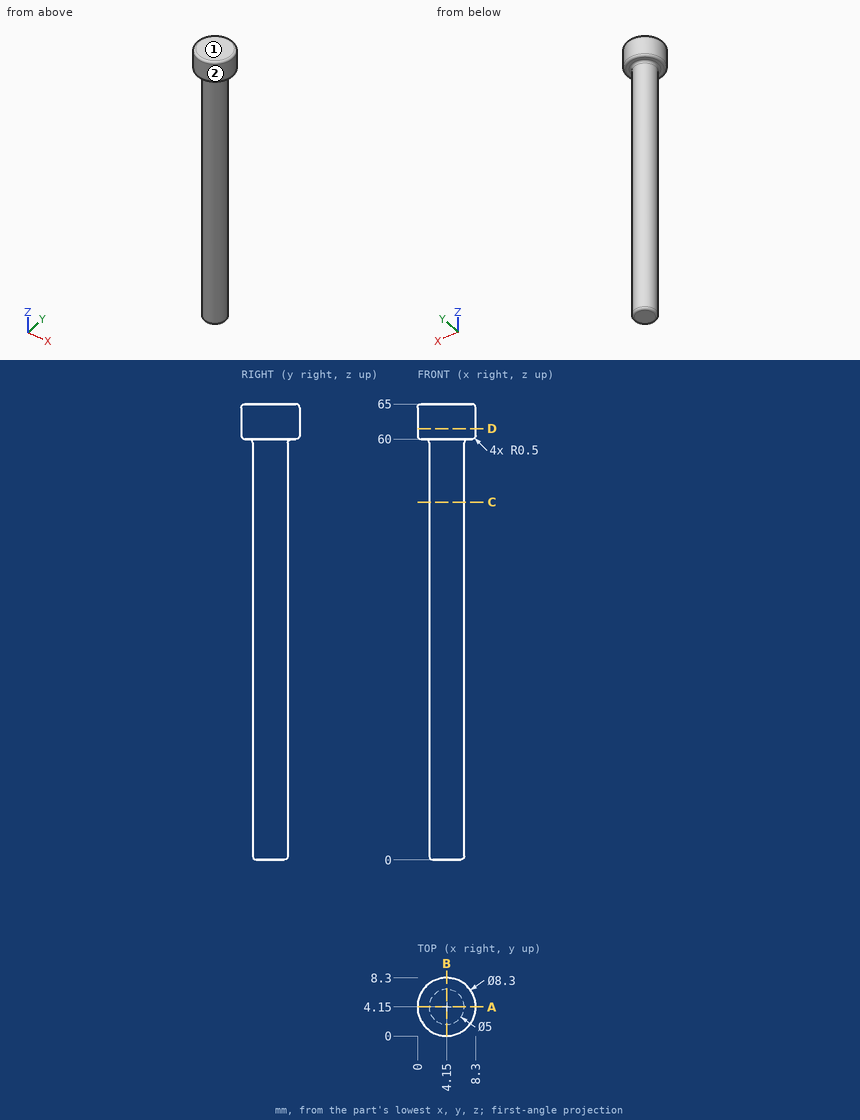
Print and shaded views of the part. All mm, measured from the part's lowest x, y and z. Coordinates: 2 decimals unless noted, no trailing zeros. Write each loop counter-clockwise with the first axis right and the second up, starting at its lowest first coordinate (ties: lowest second). Pieces come first, ordered by that corner, then holes. Notation, with made-up numbers: (-35.75, -33) -> (12.25, -33) arc R33 cw to (12.25, 1) -> close; hole circle Ø1 at (24.5, 79). An arc over 180 degrees is marked (long way). Use CSV: the item, a comma, the result in double quotes. Start each with the question number.
Q1. Drill centre lines: probe 1 along Z at (x, y) = (2.75, 7.5); probe 2 along X at (y, z) = (4, 20); probe 3 along X at (y, z) = (5.5, 20.5). Where is each one in solid material? Low to high.
Q2. Flat gauge pins, fed straight in: pin 1 Ø4 at (y, z) = (3, 42.5) entering from +X; pin 2 Ø2 at (x, z) = (4, 29.5) entering from -Y; pin 3 Ø4 at (y, z) = (7, 18.5) entering from -X. Where does each tip first touch, or does it go through?
Q3. Cut at C-C, the plane z = 51. List the corners of the cut face in (x, y), then the cut area to 3 significant figures.
Q4. Pull direction Z, two halves, no side cores. Call the marked faces 1 and 2: released by +Z, released by -Z, zero draft, split by the parting line, or undercut.
Q5. Cut at A-A, the plane y = 4.15. List the corners of the cut face in (x, z), then the cut area to 3 significant figures.
Q6. Cut at D-D, the plane z = 61.5. List the corners of the cut face in (x, y), then the cut area to 3 significant figures.
Checked values:
1,probe 1,"z = 60 to 65"
1,probe 2,"x = 1.65 to 6.65"
1,probe 3,"x = 2.05 to 6.25"
2,pin 1,"stops at x = 6.65"
2,pin 2,"stops at y = 1.65"
2,pin 3,"stops at x = 1.8"
3,outline,"circle Ø5 at (4.15, 4.15)"
3,area,"19.6 mm²"
4,face 1,"released by +Z"
4,face 2,"zero draft"
5,outline,"(0, 60.5) arc R0.5 ccw to (0.5, 60) -> (1.15, 60) arc R0.5 cw to (1.65, 59.5) -> (1.65, 0.5) arc R0.5 ccw to (2.15, 0) -> (6.15, 0) arc R0.5 ccw to (6.65, 0.5) -> (6.65, 59.5) arc R0.5 cw to (7.15, 60) -> (7.8, 60) arc R0.5 ccw to (8.3, 60.5) -> (8.3, 64.5) arc R0.5 ccw to (7.8, 65) -> (0.5, 65) arc R0.5 ccw to (0, 64.5) -> close"
5,area,"341 mm²"
6,outline,"circle Ø8.3 at (4.15, 4.15)"
6,area,"54.1 mm²"
